Check sheet for the modelled part. Datum: model origin and axes. Units: mm. Round coordinates to 2 decimals unless told otherwise and drop trailing zeros. Write each loop counter-clockwise with the first axis right and the second up, starting at its lowest first coordinate (ties: lowest second). Pieces come first, ordered by that corner, then holes. Notation, with made-up numbers: (11, 69) -> (34, 69) arc R15 ccw to (34, 93) -> close; hole circle Ø4 at (-12, 8). An arc over 180 degrees is marked (long way). One line per item, written item: value.
from build123d import *

# Parameters (mm, degrees)
SKETCH_1_R          = 1.35
SKETCH_1_W          = 10
SKETCH_1_H          = 3
SKETCH_1_W_2        = 3
SKETCH_1_H_2        = 6
SKETCH_1_W_3        = 2.381
SKETCH_1_H_3        = 1.694
SKETCH_1_W_4        = 2.327
SKETCH_1_H_4        = 1.693
SKETCH_1_W_5        = 22.999
SKETCH_1_H_5        = 12.401
SKETCH_1_W_6        = 15
EXTRUDE_1_DEPTH     = 3
SKETCH_2_R          = 1.6
CUT_EXTRUDE_1_DEPTH = 55.763647529


with BuildPart() as part:
    # 草图1 → 凸台-拉伸1 (new body)
    with BuildSketch(Plane(origin=(0, 0, 0), x_dir=(-1, 0, 0), z_dir=(0, 0, -1))):
        with BuildLine():
            Line((28.933183464, 3), (28.933183464, 41.999))
            ThreePointArc((28.933183464, 41.999), (28.054503808, 44.120320344), (25.933183464, 44.999))
            Line((25.933183464, 44.999), (-28.066816536, 44.999))
            ThreePointArc((-28.066816536, 44.999), (-30.18813688, 44.120320344), (-31.066816536, 41.999))
            Line((-31.066816536, 41.999), (-31.066816536, 3))
            ThreePointArc((-31.066816536, 3), (-30.18813688, 0.878679656), (-28.066816536, 0))
            Line((-28.066816536, 0), (25.933183464, 0))
            ThreePointArc((25.933183464, 0), (28.054503808, 0.878679656), (28.933183464, 3))
        make_face()
        with Locations(Location((-26.567767322, 12.499, 0), (0, 0, 180))):
            Circle(SKETCH_1_R, mode=Mode.SUBTRACT)
        with Locations(Location((-10.567816536, 23.43, 0), (0, 0, 180))):
            Circle(SKETCH_1_R, mode=Mode.SUBTRACT)
        with Locations(Location((24.432183464, 12.499, 0), (0, 0, 180))):
            Circle(SKETCH_1_R, mode=Mode.SUBTRACT)
        with Locations(Location((-10.567816536, 42.429, 0), (0, 0, 180))):
            Circle(SKETCH_1_R, mode=Mode.SUBTRACT)
        with Locations((16.432183464, 4.499)):
            Rectangle(SKETCH_1_W, SKETCH_1_H, mode=Mode.SUBTRACT)
        with Locations((24.433183464, 5.999)):
            Rectangle(SKETCH_1_W_2, SKETCH_1_H_2, mode=Mode.SUBTRACT)
        with Locations((24.433183464, 18.999)):
            Rectangle(SKETCH_1_W_2, SKETCH_1_H_2, mode=Mode.SUBTRACT)
        with Locations((18.298683464, 30.257)):
            Rectangle(SKETCH_1_W_3, SKETCH_1_H_3, mode=Mode.SUBTRACT)
        with Locations((18.271683464, 35.4965)):
            Rectangle(SKETCH_1_W_4, SKETCH_1_H_4, mode=Mode.SUBTRACT)
        with Locations((-10.567316536, 32.9995)):
            Rectangle(SKETCH_1_W_5, SKETCH_1_H_5, mode=Mode.SUBTRACT)
        with Locations((-16.067816536, 4.499)):
            Rectangle(SKETCH_1_W_6, SKETCH_1_H, mode=Mode.SUBTRACT)
        with Locations((-26.566816536, 5.999)):
            Rectangle(SKETCH_1_W_2, SKETCH_1_H_2, mode=Mode.SUBTRACT)
        with Locations((-26.566816536, 18.999)):
            Rectangle(SKETCH_1_W_2, SKETCH_1_H_2, mode=Mode.SUBTRACT)
    extrude(amount=-EXTRUDE_1_DEPTH)

    # 草图2 → 切除-拉伸1 (cut, through all)
    with BuildSketch(Plane.XY.offset(3)):
        with Locations((-24.432183464, 12.499)):
            Circle(SKETCH_2_R)
        with Locations((26.567767322, 12.499)):
            Circle(SKETCH_2_R)
    extrude(amount=-CUT_EXTRUDE_1_DEPTH, mode=Mode.SUBTRACT)


solid = part.part
Item 1: Sectioned sample at D-D on x = 27. Enter the section's corners in (y, z), and give its area (3 significant figures).
Answer:
outline: (0, 0) -> (3, 0) -> (3, 3) -> (0, 3) -> close; (9, 0) -> (10.96, 0) -> (10.96, 3) -> (9, 3) -> close; (14.04, 0) -> (16, 0) -> (16, 3) -> (14.04, 3) -> close; (22, 0) -> (45, 0) -> (45, 3) -> (22, 3) -> close
area: 89.8 mm^2
Item 2: Sectioned sample at C-C on y = 20. Enter the section's corners in (x, z), and give its area (3 significant figures).
Answer:
outline: (-28.93, 0) -> (-25.93, 0) -> (-25.93, 3) -> (-28.93, 3) -> close; (-22.93, 0) -> (25.07, 0) -> (25.07, 3) -> (-22.93, 3) -> close; (28.07, 0) -> (31.07, 0) -> (31.07, 3) -> (28.07, 3) -> close
area: 162 mm^2
Item 3: Depth check by flat-ended pin: P1, Ø4, axis at x = 26.57, y = 12.5, coming from the +Z side. Enter the tip coordinate at first touch or a pass-through.
Answer:
P1: stops at z = 3
Item 4: Sectioned sample at B-B on x = -18. Enter the section's corners in (y, z).
Answer:
outline: (0, 0) -> (3, 0) -> (3, 3) -> (0, 3) -> close; (6, 0) -> (29.41, 0) -> (29.41, 3) -> (6, 3) -> close; (31.1, 0) -> (34.65, 0) -> (34.65, 3) -> (31.1, 3) -> close; (36.34, 0) -> (45, 0) -> (45, 3) -> (36.34, 3) -> close
Item 5: Sectioned sample at A-A on y = 38.5. Enter the section's corners in (x, z), and give its area (3 significant figures).
Answer:
outline: (-28.93, 0) -> (-0.93, 0) -> (-0.93, 3) -> (-28.93, 3) -> close; (22.07, 0) -> (31.07, 0) -> (31.07, 3) -> (22.07, 3) -> close
area: 111 mm^2
Item 6: Thickness scan on line 1 (X direction, y = 36, z = 1.55); line 2 (X direction, y = 18, z = 1.85); line 3 (Y direction, x = 9, z = 2.4). Record the ranges inside material, lowest first.
Answer:
line 1: x = -28.93 to -19.44, -17.11 to -0.93, 22.07 to 31.07
line 2: x = -28.93 to -25.93, -22.93 to 25.07, 28.07 to 31.07
line 3: y = 0 to 3, 6 to 26.8, 39.2 to 45
